Part model, mm, in its own coordinate system. A direction names the side the tool comes from. Coordinates: 2 decimals unless noted, no trailing zeros. Order: outer loops, then holes, each group sorted by start corner. A loop starts at its lowest first (then second) coordinate and runs counter-clockwise, first axis right, second up. Notation, with made-up numbers: M 45,29.25 L 89,29.25 A17 cw 89,41.25 Z; hole C 19.25,69.5 d4. An arc over 180 degrees is marked long. Answer in a Markdown table with one row per item. Add a question column.
from build123d import *

# Parameters (mm, degrees)
F1_DEPTH = 304.8
F3_DEPTH = 25.4
F4_R     = 6.35
F5_DEPTH = 25.401
F6_R     = 12.7
F7_DEPTH = 101.601


with BuildPart() as f1:
    # F0 (on Front) → F1 (new body)
    with BuildSketch(Plane.XZ):
        with BuildLine():
            ThreePointArc((-25.4, 25.4), (0, 50.8), (25.4, 25.4))
            Line((25.4, 25.4), (25.4, 0))
            Line((25.4, 0), (101.6, 0))
            ThreePointArc((101.6, 0), (0, 101.6), (-101.6, 0))
            Line((-101.6, 0), (-25.4, 0))
            Line((-25.4, 0), (-25.4, 25.4))
        make_face()
        Polygon((101.6, 0), (25.4, 0), (0, 0), (-25.4, 0), (-101.6, 0), (-101.6, -50.8), (101.6, -50.8), align=None)
    extrude(amount=F1_DEPTH)

    # F2 (on face) → F3 (join)
    with BuildSketch(Plane(origin=(0, 0, 0), x_dir=(-1, 0, 0), z_dir=(0, 1, 0))):
        with BuildLine():
            Line((101.6, -50.8), (101.6, 0))
            ThreePointArc((101.6, 0), (0, 101.6), (-101.6, 0))
            Line((-101.6, 0), (-101.6, -50.8))
            Line((-101.6, -50.8), (101.6, -50.8))
        make_face()
    extrude(amount=F3_DEPTH)

    # F4 (on Front) → F5 (cut, through all)
    with BuildSketch(Plane.XZ):
        with Locations((0, 25.4)):
            Circle(F4_R)
    extrude(amount=-F5_DEPTH, mode=Mode.SUBTRACT)

    # F6 (on Right) → F7 (cut, through all)
    with BuildSketch(Plane.YZ):
        with Locations((-25.4, 25.4)):
            Circle(F6_R)
    extrude(amount=-F7_DEPTH, mode=Mode.SUBTRACT)


solid = f1.part
(1) Slice it at A-A (x = 0). List the corners of the cut face in (y, z).
(2) Wall check: line 1 (Z direction, x = 0, y = 5); line 2 (Y direction, x = -47, z = 25); line 3 (Z direction, x = -37.5, y = -25.4). Give the ranges that are in metal, low to high.
(3) 3-axis set-ups, long thin cutter, end or side, ignore diameter. For faces 4 (the cylindrical face through (-60.848, -19.54, 14.133)), 5 (the flat face through (25.4, -150, 13)), 6 (the flat face through (-101.6, -142, -26)): which of +Z, -Z, +X, -X, +Y, -Y reach the whole face in a straight line?
(4) Pull direction Z, two halves, no side cores. Call faces 1 (the cylindrical face through (-0.559, -150.266, 50.794)), 2 (the flat face through (-1, -304.8, -7)), 3 (the flat face through (1, -142, -50.8)): pulls with the +Z half, pulls with the -Z half, needs draft (parallel to the pull), parting line crosses it, or undercut.
(5) Slice it at D-D (y = -25.4). List the corners of the cut face in (x, z).
(6) Drop flat-ended pins along their axis: P1, Ø7.5, axis at y = -208.5, z = 15, coming from the +X side; P2, Ø5, axis at y = -92, z = 86, coming from the -X side; P3, Ø15, axis at y = -25.4, z = 25.4, coming from the +X side. Give the stop position or say it passes through.
(7) Slice it at C-C (x = -55). List the corners of the cut face in (y, z), and give its area (3 significant figures).
(8) Slice it at B-B (y = -77). List the corners of the cut face in (x, z), and give its area (3 significant figures).
Computed:
| question | item | result |
|---|---|---|
| 1 | outline | M -304.8,-50.8 L 25.4,-50.8 L 25.4,19.05 L 0,19.05 L 0,0 L -304.8,0 Z; M -304.8,50.8 L 0,50.8 L 0,31.75 L 25.4,31.75 L 25.4,101.6 L -304.8,101.6 Z |
| 2 | line 1 | z = -50.8 to 19.05, 31.75 to 101.6 |
| 2 | line 2 | y = -304.8 to -38.09, -12.71 to 25.4 |
| 2 | line 3 | z = -50.8 to 12.7, 38.1 to 94.43 |
| 3 | face 4 | -X |
| 3 | face 5 | -Y |
| 3 | face 6 | +Z, -Z, -X, +Y, -Y |
| 4 | face 1 | undercut |
| 4 | face 2 | needs draft |
| 4 | face 3 | pulls with the -Z half |
| 5 | outline | M -101.6,-50.8 L 101.6,-50.8 L 101.6,0 A101.6 ccw -94.19,38.1 L -22,38.1 A25.4 cw 25.4,25.4 L 25.4,0 L -25.4,0 L -25.4,12.7 L -100.8,12.7 A101.6 ccw -101.6,0 Z |
| 6 | P1 | stops at x = 100.98 |
| 6 | P2 | stops at x = -57.88 |
| 6 | P3 | stops at x = 100.01 |
| 7 | outline | M -304.8,-50.8 L 25.4,-50.8 L 25.4,85.43 L -304.8,85.43 Z; hole C -25.4,25.4 d25.4 |
| 7 | area | 44,500 mm^2 |
| 8 | outline | M -101.6,-50.8 L 101.6,-50.8 L 101.6,0 A101.6 ccw -101.6,0 Z; hole M -25.4,0 L 25.4,0 L 25.4,25.4 A25.4 ccw -25.4,25.4 Z |
| 8 | area | 24,200 mm^2 |
